Read the model definition and answer for the solid it produces. Units are mm, in the model's axes. Face numbers are marked on the shaded views. A direction names the side the tool comes from. Coordinates: 2 decimals unless noted, no trailing zeros. Order: outer loops, then holes, each group sorted by start corner. A loop starts at its lowest first (then second) coordinate and runs counter-clockwise, first axis right, second up. Notation, with made-up numbers: (55, -30) - (80, -30) arc R19 cw to (80, -8) - close; hole circle Ø7 at (28, 61.25). An arc over 180 degrees is marked (long way). Write item = value, one per line.
from build123d import *

# Parameters (mm, degrees)
BOSS_EXTRUDE1_DEPTH = 38
SKETCH2_W           = 43
SKETCH2_H           = 43
BOSS_EXTRUDE2_DEPTH = 3
SKETCH3_R           = 2
SKETCH3_R_2         = 12.25
CUT_EXTRUDE1_DEPTH  = 10
SKETCH4_R           = 2.5
CUT_EXTRUDE2_DEPTH  = 10
SKETCH5_W           = 20
SKETCH5_H           = 20
SKETCH5_R           = 2.5
BOSS_EXTRUDE3_DEPTH = 4
FILLET1_R           = 1


with BuildPart() as part:
    # Sketch1 → Boss-Extrude1 (new body)
    with BuildSketch(Plane(origin=(0, 0, 0), x_dir=(1, 0, 0), z_dir=(0, 1, 0))):
        Polygon((0, 0), (0, 34), (-20, 34), (-20, 38), (4, 38), (4, -5), (47, -5), (47, -9), (0, -9), align=None)
    extrude(amount=BOSS_EXTRUDE1_DEPTH)

    # Sketch2 → Boss-Extrude2 (add)
    with BuildSketch(Plane(origin=(0, 38, 0), x_dir=(1, 0, 0), z_dir=(0, 1, 0))):
        with Locations((25.5, 16.5)):
            Rectangle(SKETCH2_W, SKETCH2_H)
    extrude(amount=-BOSS_EXTRUDE2_DEPTH)

    # Sketch3 → Cut-Extrude1 (cut)
    with BuildSketch(Plane(origin=(0, 35, 0), x_dir=(-1, 0, 0), z_dir=(0, -1, 0))):
        with Locations((-40.5, 31.5)):
            Circle(SKETCH3_R)
        with Locations((-9.5, 31.5)):
            Circle(SKETCH3_R)
        with Locations((-9.5, 0.5)):
            Circle(SKETCH3_R)
        with Locations((-40.5, 0.5)):
            Circle(SKETCH3_R)
        with Locations((-25, 16)):
            Circle(SKETCH3_R_2)
    extrude(amount=-CUT_EXTRUDE1_DEPTH, mode=Mode.SUBTRACT)

    # Sketch4 → Cut-Extrude2 (cut)
    with BuildSketch(Plane.XY.offset(-34)):
        with Locations((-10, 10)):
            Circle(SKETCH4_R)
        with Locations((-10, 28)):
            Circle(SKETCH4_R)
    extrude(amount=-CUT_EXTRUDE2_DEPTH, mode=Mode.SUBTRACT)

    # Sketch5 → Boss-Extrude3 (add)
    with BuildSketch(Plane.ZY):
        with Locations((19, 10)):
            Rectangle(SKETCH5_W, SKETCH5_H)
        with Locations((16, 10)):
            Circle(SKETCH5_R, mode=Mode.SUBTRACT)
        with Locations((24, 10)):
            Circle(SKETCH5_R, mode=Mode.SUBTRACT)
    extrude(amount=-BOSS_EXTRUDE3_DEPTH)

    # Fillet1
    fillet1_edges = [part.edges().sort_by_distance(p)[0] for p in [
        (4, 17.5, -38),
        (4, 10, 9),
    ]]
    fillet(fillet1_edges, radius=FILLET1_R)


solid = part.part
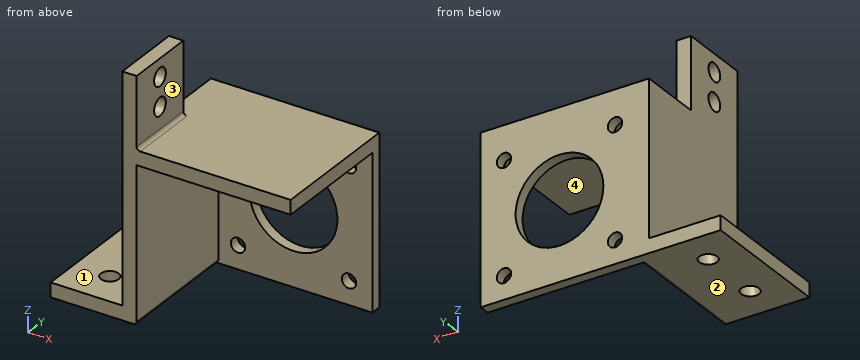
1) Straight lines are drawn through the part: line 1 along X through (y, z) = (35.95, -31.5); line 2 along Y through (x, z) = (-10, -35.3); line 3 along Z through (x, y) = (9.5, 36.1). For each, find the intervals that lie inside material, in ascending order. Write a range as from..to.
Returned:
line_1 = 0..7.5, 11.5..38.5, 42.5..47
line_2 = 0..7.5, 12.5..25.5, 30.5..38
line_3 = -38..-33.5, -29.5..-2.5, 1.5..9
2) For the marked faces 1, 2, 3 and 4, determine the directions among +Z, -Z, +X, -X, +Y, -Y from which every point of the face is accessible in a straight line to the end or side of a thin tool.
Returned:
face_1 = +Z, -X, +Y, -Y
face_2 = -Z, +X, -X, +Y, -Y
face_3 = +Z, +X, +Y, -Y
face_4 = -Z, +X, -Y
3) The part is cut by section D-D (z = -31.5). Determine the outline of the cut face in (x, y).
Returned:
outline = (0, 0) - (4, 0) - (4, 35) - (7.5, 35) - (7.5, 38) - (0, 38) - close; (11.5, 35) - (38.5, 35) - (38.5, 38) - (11.5, 38) - close; (42.5, 35) - (47, 35) - (47, 38) - (42.5, 38) - close
4) The part is cut by section B-B (z = -16). Determine the outline of the cut face in (x, y), and give its area (4 significant figures).
Returned:
outline = (0, 0) - (4, 0) - (4, 35) - (12.75, 35) - (12.75, 38) - (0, 38) - close; (37.25, 35) - (47, 35) - (47, 38) - (37.25, 38) - close
area = 207.5 mm^2
5) The part is cut by section A-A (y = 28). Determine the outline of the cut face in (x, z).
Returned:
outline = (-20, -38) - (-12.5, -38) - (-12.5, -34) - (-20, -34) - close; (-7.5, -38) - (3, -38) arc R1 ccw to (4, -37) - (4, 5) - (47, 5) - (47, 9) - (0, 9) - (0, -34) - (-7.5, -34) - close
6) Flat-ended cylindrical pins translate along their axes: pin 1 Ø17.5 at (y, z) = (17, -14.5) entering from +X; pin 2 Ø10 at (x, z) = (10.5, -8.5) entering from -Y; pin 3 Ø10 at (x, y) = (23.5, 26.5) entering from -Z. Find the tip coordinate at first contact, or state that the pin passes through.
Returned:
pin_1 = 4
pin_2 = 35
pin_3 = 5
7) The part is cut by section C-C (x = -10). Determine the outline of the cut face in (y, z).
Returned:
outline = (0, -38) - (7.5, -38) - (7.5, -34) - (0, -34) - close; (12.5, -38) - (25.5, -38) - (25.5, -34) - (12.5, -34) - close; (30.5, -38) - (38, -38) - (38, -34) - (30.5, -34) - close
